from build123d import *

# Parameters (mm, degrees)
F0_R     = 4
F0_R_2   = 2
F5_DEPTH = 0.5
F2_R     = 2.5
F2_R_2   = 1.5
F6_DEPTH = 2.62
F4_R     = 4
F4_R_2   = 2
F7_DEPTH = 0.5


with BuildPart() as f5:
    # F0 (on Top) → F5 (new body, symmetric)
    with BuildSketch(Plane.XY):
        Circle(F0_R)
        Circle(F0_R_2, mode=Mode.SUBTRACT)
    extrude(amount=F5_DEPTH, both=True)

    # F2 (on offset) → F6 (join, symmetric)
    with BuildSketch(Plane.XY.offset(2.62)):
        Circle(F2_R)
        Circle(F2_R_2, mode=Mode.SUBTRACT)
    extrude(amount=F6_DEPTH, both=True)

    # F4 (on offset) → F7 (join, symmetric)
    with BuildSketch(Plane.XY.offset(5.24)):
        Circle(F4_R)
        Circle(F4_R_2, mode=Mode.SUBTRACT)
    extrude(amount=F7_DEPTH, both=True)


solid = f5.part
Work out the finished part from the listing and answer in its coordinate system (mm). A direction names the side the tool comes from. Round coordinates to 2 decimals unless told otherwise and drop trailing zeros. Loops run counter-clockwise (first coordinate to the right, second up) from the corner with the lowest first, then second, coordinate; pieces in that order, holes last. Notation, with made-up numbers: (50, 15.25) - (91, 15.25) arc R12 cw to (91, 31.25) - close; hole circle Ø7 at (-11.75, 78). An arc over 180 degrees is marked (long way). Use one line per item in the form item = value. Start each with the question number.
(1) Determine the mould class of faces 1 (the face through (-0.434, -1.952, 5.486)), 2 (the face through (-0.54, -2.44, 2.65)), 3 (the face through (-2, -1, 5.74)) for opening direction Y: +Y half, -Y half, draft (parallel to the pull), parting line (faces both ways), or undercut.
(2) Find section C-C on z = 3.25. Determine the outline of the cut face in (x, y).
(3) Find section A-A on y = 0. Determine the outline of the cut face in (x, z).
(4) Find section D-D on y = -3. Determine the outline of the cut face in (x, z).
(5) Consider line 1 (Z direction, x = -1.75, y = -3.25); line 2 (Y direction, x = 0, z = -0.3); line 3 (Y direction, x = 0, z = 1.6). Determine where each line is inside the solid, lowest interval first.
(6) Flat-ended cylindrical pins translate along their axes: P1, Ø1.5, axis at y = -2.5, z = 2, coming from the -X side; P2, Ø3.5, axis at x = 0, y = 0, coming from the +Z side; P3, Ø1.2, axis at x = 0, y = -1, coming from the -Z side. Find the tip coordinate at first contact, or state that the pin passes through.
(7) Which of the six approach directions +Z, -Z, +X, -X, +Y, -Y give full straight-line access (tool end or side, diameter ignored) to faces 4 (the face through (-0.434, -1.952, -0.254)), 5 (the face through (-0.867, -3.905, 0.007)), 6 (the face through (2, 2, 4.74))?
Answer list:
q1.face_1 = undercut
q1.face_2 = parting line
q1.face_3 = draft
q2.outline = circle Ø5 at (0, 0); hole circle Ø3 at (0, 0)
q3.outline = (-4, -0.5) - (-2, -0.5) - (-2, 0) - (-1.5, 0) - (-1.5, 5.24) - (-2, 5.24) - (-2, 5.74) - (-4, 5.74) - (-4, 4.74) - (-2.5, 4.74) - (-2.5, 0.5) - (-4, 0.5) - close; (1.5, 0) - (2, 0) - (2, -0.5) - (4, -0.5) - (4, 0.5) - (2.5, 0.5) - (2.5, 4.74) - (4, 4.74) - (4, 5.74) - (2, 5.74) - (2, 5.24) - (1.5, 5.24) - close
q4.outline = (-2.65, -0.5) - (2.65, -0.5) - (2.65, 0.5) - (-2.65, 0.5) - close; (-2.65, 4.74) - (2.65, 4.74) - (2.65, 5.74) - (-2.65, 5.74) - close
q5.line_1 = -0.5 to 0.5, 4.74 to 5.74
q5.line_2 = -4 to -2, 2 to 4
q5.line_3 = -2.5 to -1.5, 1.5 to 2.5
q6.P1 = -1.79
q6.P2 = 5.24
q6.P3 = 0
q7.face_4 = -Z
q7.face_5 = +Z, -Z
q7.face_6 = none
